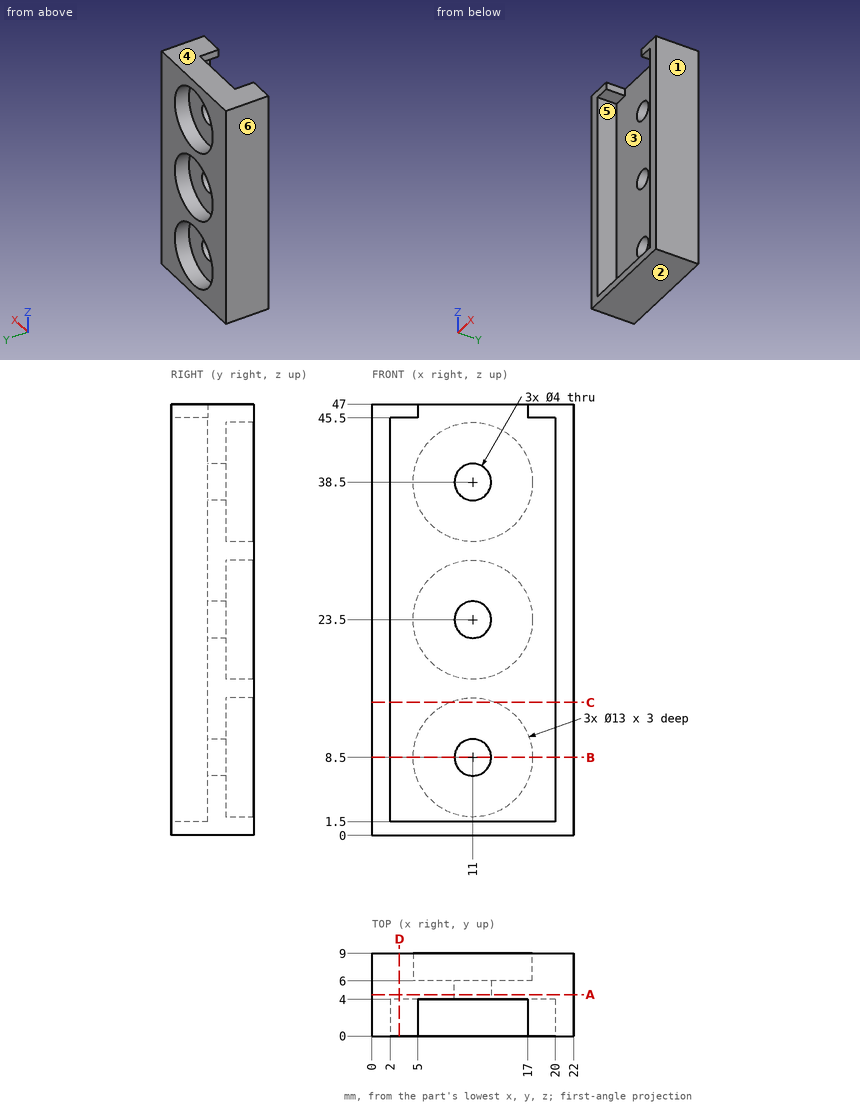
Study the drawing (mm; zero at the part's minimum x, y, z) and answer. A direction names the side the tool comes from. Coordinates: 2 decimals unless noted, no trailing zeros. Write each loop counter-clockwise with the first axis right and the second up, starting at its lowest first coordinate (ties: lowest second). Pieces come first, ordered by that corner, then holes. Notation, with made-up numbers: (66.25, 66) - (117.25, 66) arc R17 ccw to (117.25, 99) - close; hole circle Ø11 at (6.25, -38). An arc over 180 degrees is marked (long way). Answer as a JSON object with one key per item and string values.
Q1. Given pin 1 Ø4.5 at (x, y) = (11.5, 1) entering from +Z; pin 2 Ø6.5 at (x, z) = (11, 38.5) entering from +Y; pin 3 Ø6.5 at (x, z) = (11, 8.5) entering from -Y, each flat-ended and moving along its own axis, determine where each tip first touches the part or whether it passes through.
Results list:
{"pin 1": "stops at z = 1.5", "pin 2": "stops at y = 6", "pin 3": "stops at y = 4"}
Q2. Find section A-A (y = 4.5). Write down the section's boundary in (x, z).
Results list:
{"outline": "(0, 0) - (22, 0) - (22, 47) - (0, 47) - close; hole circle Ø4 at (11, 8.5); hole circle Ø4 at (11, 23.5); hole circle Ø4 at (11, 38.5)"}
Q3. Which of the six approach directions +Z, -Z, +X, -X, +Y, -Y give full straight-line access (tool end or side, diameter ignored) to the marked faces 5 and 6?
Results list:
{"face 5": "-Y", "face 6": "+Z, -Z, -X, +Y, -Y"}
Q4. For a pull along Z with two mould halves and no side action, classify the marked faces 1, 2, 3 and 4 as pulls with the +Z half, pulls with the -Z half, needs draft (parallel to the pull), parting line crosses it, or undercut.
Results list:
{"face 1": "needs draft", "face 2": "pulls with the -Z half", "face 3": "undercut", "face 4": "pulls with the +Z half"}
Q5. Find section B-B (z = 8.5). Write down the section's boundary in (x, y), plus the area to 3 significant figures.
Results list:
{"outline": "(0, 0) - (2, 0) - (2, 4) - (9, 4) - (9, 6) - (4.5, 6) - (4.5, 9) - (0, 9) - close; (13, 4) - (20, 4) - (20, 0) - (22, 0) - (22, 9) - (17.5, 9) - (17.5, 6) - (13, 6) - close", "area": "79.0 mm^2"}
Q6. Find section C-C (z = 14.5). Write down the section's boundary in (x, y).
Results list:
{"outline": "(0, 0) - (2, 0) - (2, 4) - (20, 4) - (20, 0) - (22, 0) - (22, 9) - (13.5, 9) - (13.5, 6) - (8.5, 6) - (8.5, 9) - (0, 9) - close"}
Q7. Find section D-D (x = 3). Write down the section's boundary in (y, z), plus the area to 3 significant figures.
Results list:
{"outline": "(0, 0) - (9, 0) - (9, 47) - (0, 47) - (0, 45.5) - (4, 45.5) - (4, 1.5) - (0, 1.5) - close", "area": "247 mm^2"}
Q8. Consider L1, parallel to Z at x = 11, y = 7.6; L2, parallel to X at y = 4.9, z = 38.5; L3, parallel to X at y = 8.4, z = 38.5. Determine where each line is inside the solid, lowest interval first. Write a range as from..to.
Results list:
{"L1": "z = 0..2, 15..17, 30..32, 45..47", "L2": "x = 0..9, 13..22", "L3": "x = 0..4.5, 17.5..22"}
